Could you check a few things on this model? Use its own coordinates, in mm. A direction names the side the tool comes from. Coordinates: 2 decimals unless noted, no trailing zeros. Write each loop counter-clockwise with the first axis right and the second up, starting at its lowest first coordinate (ties: lowest second). Pieces come first, ordered by that corner, then holes.
Item 1: Which directions (+Z, -Z, +X, -X, +Y, -Y) give clear straight access to the entire face, cutting with the end or side of a thin tool? Please do faces 4 (the flat face through (2.74, 13, -2)), 5 (the flat face through (8, 14, 0)), 6 (the cylindrical face through (8.893, 6.519, 1.521)).
Item 2: I want a section at B-B on x = 32.25. Please give me the cut outline in (y, z), then the cut area to 3 significant figures.
Item 3: For P1, Ø1.4, axis at x = 19.5, z = -3, coming from the -Y side; P2, Ø2, axis at x = 4.5, y = 17, coming from the -Z side; P3, Ø1.4, axis at x = 12.5, z = -1.5, coming from the +Y side; P4, Ø1, axis at x = 32, y = 27.5, coming from the -Z side, each with a flat end and sliding along its axis, tell me the tip position at first contact or that it passes through.
Item 4: Thinking about a two-plate mould opening in Y: for faces 1 (the flat face through (10.026, 28.151, 1.479)), 2 (the flat face through (13, 2.09, -2)), 3 (the flat face through (24, 9, 0)), which applies, +Y half, -Y half, draft (parallel to the pull), parting line (faces both ways), or undercut?
Item 5: I want a section at C-C on x = 23.75. Please give me the cut outline in (y, z), then the cut area to 3 significant figures.
Item 6: If I drill on probe 1 along Y at (x, z) = (23.5, -2.25); probe 2 along Y at (x, z) = (22.5, 1.75); probe 3 along Z at (x, y) = (13.5, 34), over which ranges is the centre line in solid material (lowest first)?
Item 7: I want a section at A-A on z = -3.5. Please give me the cut outline in (x, y), then the cut area to 3 significant figures.
Item 8: I want a section at D-D on z = 2. Please give me the cut outline in (x, y).
from build123d import *

# Parameters (mm, degrees)
SKETCH004_W      = 32.8
SKETCH004_H      = 22.66
SKETCH004_W_2    = 22.4
SKETCH004_H_2    = 12.76
EXTRUDE002_DEPTH = 4.8
SKETCH_R         = 3.15
EXTRUDE001_DEPTH = 5
SKETCH003_R      = 1.94
SKETCH003_R_2    = 6.38
EXTRUDE_DEPTH    = 3
FILLET_R         = 15


with BuildPart() as extrude002:
    # Sketch004 → Extrude002 (new body)
    with BuildSketch(Plane.XY):
        with Locations((13.69, 13.42)):
            Rectangle(SKETCH004_W, SKETCH004_H)
        with Locations((13.94, 13.42)):
            Rectangle(SKETCH004_W_2, SKETCH004_H_2, mode=Mode.SUBTRACT)
    extrude(amount=-EXTRUDE002_DEPTH)


with BuildPart() as extrude001:
    # Sketch (on Face5 of Fillet) → Extrude001 (new body, symmetric)
    with BuildSketch(Plane.XY.offset(3)):
        with Locations((12.283935, 13.42)):
            Circle(SKETCH_R)
    extrude(amount=EXTRUDE001_DEPTH, both=True)


with BuildPart() as fusion:
    # Sketch003 → Extrude (new body)
    with BuildSketch(Plane.XY):
        Polygon((0, 0), (13, 36.5), (43, 36.5), (56, 0), align=None)
        with Locations((23.75, 30.714505)):
            Circle(SKETCH003_R, mode=Mode.SUBTRACT)
        with Locations((32.25, 30.714505)):
            Circle(SKETCH003_R, mode=Mode.SUBTRACT)
        with Locations((37.24, 13.42)):
            Circle(SKETCH003_R, mode=Mode.SUBTRACT)
        with Locations((18.76, 13.42)):
            Circle(SKETCH003_R_2, mode=Mode.SUBTRACT)
    extrude(amount=EXTRUDE_DEPTH)

    # Fillet
    fillet_edges = [fusion.edges().sort_by_distance(p)[0] for p in [
        (0, 0, 1.5),
        (56, 0, 1.5),
    ]]
    fillet(fillet_edges, radius=FILLET_R)

    # Cut: cut Extrude001
    add(extrude001.part, mode=Mode.SUBTRACT)

    # Fusion: union Extrude002
    add(extrude002.part)


solid = fusion.part
Response values:
1. face 4: +Z, -Z
1. face 5: -Z
1. face 6: +Z, -X
2. outline: (0, 0) - (28.77, 0) - (28.77, 3) - (0, 3) - close; (32.65, 0) - (36.5, 0) - (36.5, 3) - (32.65, 3) - close
2. area: 97.9 mm2
3. P1: stops at y = 2.09
3. P2: passes through
3. P3: stops at y = 24.75
3. P4: stops at z = 0
4. face 1: +Y half
4. face 2: -Y half
4. face 3: undercut
5. outline: (0, 0) - (2.09, 0) - (2.09, -4.8) - (7.04, -4.8) - (7.04, 0) - (9.44, 0) - (9.44, 3) - (0, 3) - close; (17.4, 0) - (19.8, 0) - (19.8, -4.8) - (24.75, -4.8) - (24.75, 0) - (28.77, 0) - (28.77, 3) - (17.4, 3) - close; (32.65, 0) - (36.5, 0) - (36.5, 3) - (32.65, 3) - close
5. area: 122 mm2
6. probe 1: y = 2.09 to 7.04, 19.8 to 24.75
6. probe 2: y = 0 to 8.25, 18.59 to 29.23, 32.2 to 36.5
6. probe 3: z = 0 to 3
7. outline: (-2.71, 2.09) - (30.09, 2.09) - (30.09, 24.75) - (-2.71, 24.75) - close; hole (2.74, 7.04) - (25.14, 7.04) - (25.14, 19.8) - (2.74, 19.8) - close
7. area: 457 mm2
8. outline: (7.13, 20.03) arc R15 ccw to (21.27, 0) - (34.73, 0) arc R15 ccw to (48.87, 20.03) - (43, 36.5) - (13, 36.5) - close; hole (13.15, 10.39) arc R6.38 ccw (long way) to (13.15, 16.45) arc R3.15 ccw (long way) to start; hole circle Ø3.88 at (23.75, 30.71); hole circle Ø3.88 at (32.25, 30.71); hole circle Ø3.88 at (37.24, 13.42)
